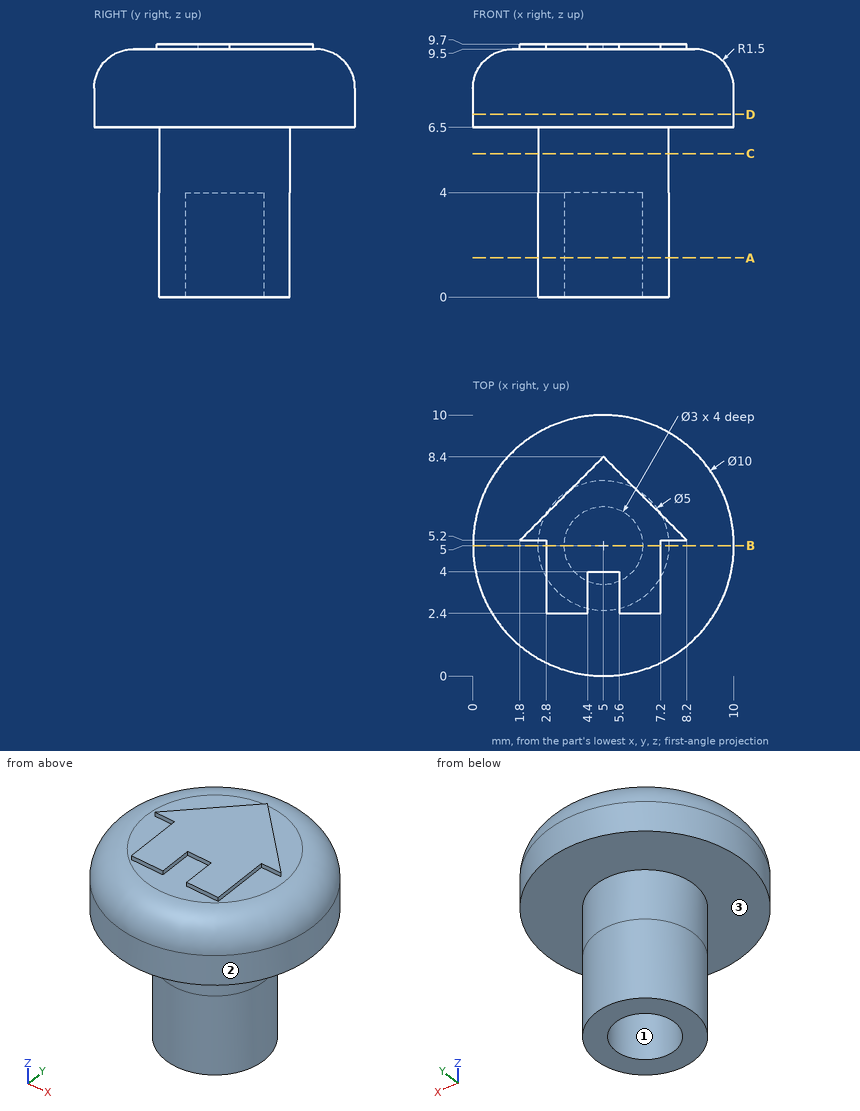
Input: dimensioned drawing with shaded views. Units: mm. Origin: part minimum x, y, z. Coordinates: 2 decimals unless noted, no trailing zeros. Order: outer loops, then holes, each group sorted by start corner. A loop starts at its lowest first (then second) coordinate and runs counter-clockwise, first axis right, second up. Notation, with made-up numbers: (69, 66.5) - (91, 66.5) arc R27 ccw to (91, 87.5) - close; hole circle Ø7 at (45.5, -8.5). An arc over 180 degrees is marked (long way). Return JSON: item names as keys, results as strings. Group by question number.
1. Cut plane D-D (z = 7). Output: boundary loops of the cut face in (x, y).
2. Pull-direction query (X, two-part tool) for the marked faces 1, 2 and 3; classes: pulls with the +X half, pulls with the -X half, needs draft (parallel to the pull), parting line crosses it, or undercut.
3. Cut plane C-C (z = 5.5). Output: boundary loops of the cut face in (x, y), plus the area to 3 significant figures.
4. Pin query (flat end, axial travel): pin 1 (3 mm diameter, centred on y = 8.5, z = 7.5, fed in from -X); pin 2 (1.5 mm diameter, centred on y = 7, z = 4.5, fed in from +X); pin 3 (2 mm diameter, centred on x = 4.5, z = 4, fed in from +Y). Return the tip coordinate at first contact, or that it passes through.
5. Cut plane B-B (y = 5). Output: boundary loops of the cut face in (x, z).
6. Material intervals for line 1 along X through (y, z) = (5, 1.95); line 2 along X through (y, z) = (7, 4.75), sorted ascending. Write a range as [from, to].
7. Cut plane A-A (z = 1.5). Output: boundary loops of the cut face in (x, y), plus the area to 3 significant figures.
Resolved:
{
 "1": {"outline": "circle Ø10 at (5, 5)"},
 "2": {"face 1": "undercut", "face 2": "parting line crosses it", "face 3": "needs draft"},
 "3": {"outline": "circle Ø5 at (5, 5)", "area": "19.6 mm²"},
 "4": {"pin 1": "stops at x = 0.42", "pin 2": "stops at x = 7.17", "pin 3": "stops at y = 7.5"},
 "5": {"outline": "(0, 6.5) - (2.5, 6.5) - (2.5, 0) - (3.5, 0) - (3.5, 4) - (6.5, 4) - (6.5, 0) - (7.5, 0) - (7.5, 6.5) - (10, 6.5) - (10, 8) arc R1.5 ccw to (8.5, 9.5) - (7.2, 9.5) - (7.2, 9.7) - (2.8, 9.7) - (2.8, 9.5) - (1.5, 9.5) arc R1.5 ccw to (0, 8) - close"},
 "6": {"line 1": "x = [2.5, 3.5], [6.5, 7.5]", "line 2": "x = [3.5, 6.5]"},
 "7": {"outline": "circle Ø5 at (5, 5); hole circle Ø3 at (5, 5)", "area": "12.6 mm²"}
}
